from build123d import *

# Parameters (mm, degrees)
SKETCH1_W           = 38.1
SKETCH1_H           = 8.382
BOSS_EXTRUDE1_DEPTH = 25.4
SKETCH2_W           = 4.3942
SKETCH2_H           = 4.3942
BOSS_EXTRUDE2_DEPTH = 25.4
SKETCH3_W           = 12.7
SKETCH3_H           = 8.382
BOSS_EXTRUDE3_DEPTH = 25.4
SKETCH4_W           = 21.5392
SKETCH4_H           = 31.75
BOSS_EXTRUDE4_DEPTH = 6.35
SKETCH5_R           = 10.7696
BOSS_EXTRUDE5_DEPTH = 25.4


with BuildPart() as part:
    # Sketch1 → Boss-Extrude1 (new body)
    with BuildSketch(Plane.XY):
        with Locations((-19.05, 4.191)):
            Rectangle(SKETCH1_W, SKETCH1_H)
    extrude(amount=BOSS_EXTRUDE1_DEPTH)

    # Sketch2 → Boss-Extrude2 (add)
    with BuildSketch(Plane.XY.offset(25.4)):
        with Locations((-35.9029, 10.5791)):
            Rectangle(SKETCH2_W, SKETCH2_H)
        with Locations((-2.1971, 10.5791)):
            Rectangle(SKETCH2_W, SKETCH2_H)
    extrude(amount=-BOSS_EXTRUDE2_DEPTH)

    # Sketch3 → Boss-Extrude3 (add)
    with BuildSketch(Plane.XY.offset(25.4)):
        with Locations((-31.75, 16.9672)):
            Rectangle(SKETCH3_W, SKETCH3_H)
        with Locations((-6.35, 16.9672)):
            Rectangle(SKETCH3_W, SKETCH3_H)
    extrude(amount=-BOSS_EXTRUDE3_DEPTH)


with BuildPart() as body_2:
    # Sketch4 → Boss-Extrude4 (new body)
    with BuildSketch(Plane(origin=(0, 0, 0), x_dir=(-1, 0, 0), z_dir=(0, 0, -1))):
        with Locations((19.05, -15.875)):
            Rectangle(SKETCH4_W, SKETCH4_H)
    extrude(amount=-BOSS_EXTRUDE4_DEPTH)

    # Sketch5 → Boss-Extrude5 (add)
    with BuildSketch(Plane(origin=(0, 0, 0), x_dir=(-1, 0, 0), z_dir=(0, 0, -1))):
        with Locations((19.05, -31.75)):
            Circle(SKETCH5_R)
    extrude(amount=-BOSS_EXTRUDE5_DEPTH)

    # Combine1: union part
    add(part.part)


solid = body_2.part
Could you check a few things on this model? Use its own coordinates, in mm. A direction names the side the tool comes from. Coordinates: 2 decimals unless noted, no trailing zeros. Order: outer loops, then holes, each group sorted by start corner. A loop starts at its lowest first (then second) coordinate and runs counter-clockwise, first axis right, second up.
Q1. Suppose I cut it at D-D on y = -15. Please give me the cut outline in (x, z).
Q2. Which directions (+Z, -Z, +X, -X, +Y, -Y) give clear straight access to the entire face, cutting with the end or side of a thin tool? Please do faces 4 (the flat face through (-4.394, 11, 13)), 5 (the cylindrical face through (-16.715, -42.264, 12.522)), 6 (the flat face through (-8.28, -16, 3)), 7 (the flat face through (-29.82, -16, 3)).
Q3. Thinking about a two-plate mould opening in X: for faces 1 (the flat face through (0, 10, 13)), 2 (the flat face through (-19, 8.382, 13)), 3 (the flat face through (-19, -12, 6.35)), which applies, released by +X, released by -X, zero draft, split by the parting line, or undercut?
Q4. Suppose I cut it at B-B on y = 14. Please give me the cut outline in (x, z), and give its area (3 significant figures).
Q5. Will these pins go through, and if not, where does the flat tip stop? pin 1 (7 mm diameter, centred on y = -12.5, z = 3, fed in from -X); pin 2 (3 mm diameter, centred on y = -15.5, z = 1.5, fed in from +X); pin 3 (8 mm diameter, centred on x = -25.5, y = -25, fed in from -Z); pin 4 (10 mm diameter, centred on x = -27, z = 5.5, fed in from -Y).
Q6. Please list where these lines run through material, in increasing order: L1, parallel to X at y = 15, z = 10.25; L2, parallel to X at y = 12, z = 3; L3, parallel to Y at x = -9.5, z = 11.
Q7. Suppose I cut it at A-A on x = -31. Please give me the cut outline in (y, z).
Q8. Suppose I cut it at C-C on x = -19.05. Please give me the cut outline in (y, z), and give its area (3 significant figures).
Answer:
1. outline: (-29.82, 0) - (-8.28, 0) - (-8.28, 6.35) - (-29.82, 6.35) - close
2. face 4: +Z, -Z
2. face 5: +Z
2. face 6: +Z, -Z, +X, -Y
2. face 7: +Z, -Z, -X, -Y
3. face 1: released by +X
3. face 2: undercut
3. face 3: zero draft
4. outline: (-38.1, 0) - (-25.4, 0) - (-25.4, 25.4) - (-38.1, 25.4) - close; (-12.7, 0) - (0, 0) - (0, 25.4) - (-12.7, 25.4) - close
4. area: 645 mm2
5. pin 1: stops at x = -29.82
5. pin 2: stops at x = -8.28
5. pin 3: stops at z = 0
5. pin 4: stops at y = -42.11
6. L1: x = -38.1 to -25.4, -12.7 to 0
6. L2: x = -38.1 to -33.71, -4.39 to 0
6. L3: y = -36.73 to -26.77, 0 to 8.38, 12.78 to 21.16
7. outline: (0, 0) - (8.38, 0) - (8.38, 25.4) - (0, 25.4) - close; (12.78, 0) - (21.16, 0) - (21.16, 25.4) - (12.78, 25.4) - close
8. outline: (-42.52, 0) - (8.38, 0) - (8.38, 25.4) - (0, 25.4) - (0, 6.35) - (-20.98, 6.35) - (-20.98, 25.4) - (-42.52, 25.4) - close
8. area: 893 mm2
